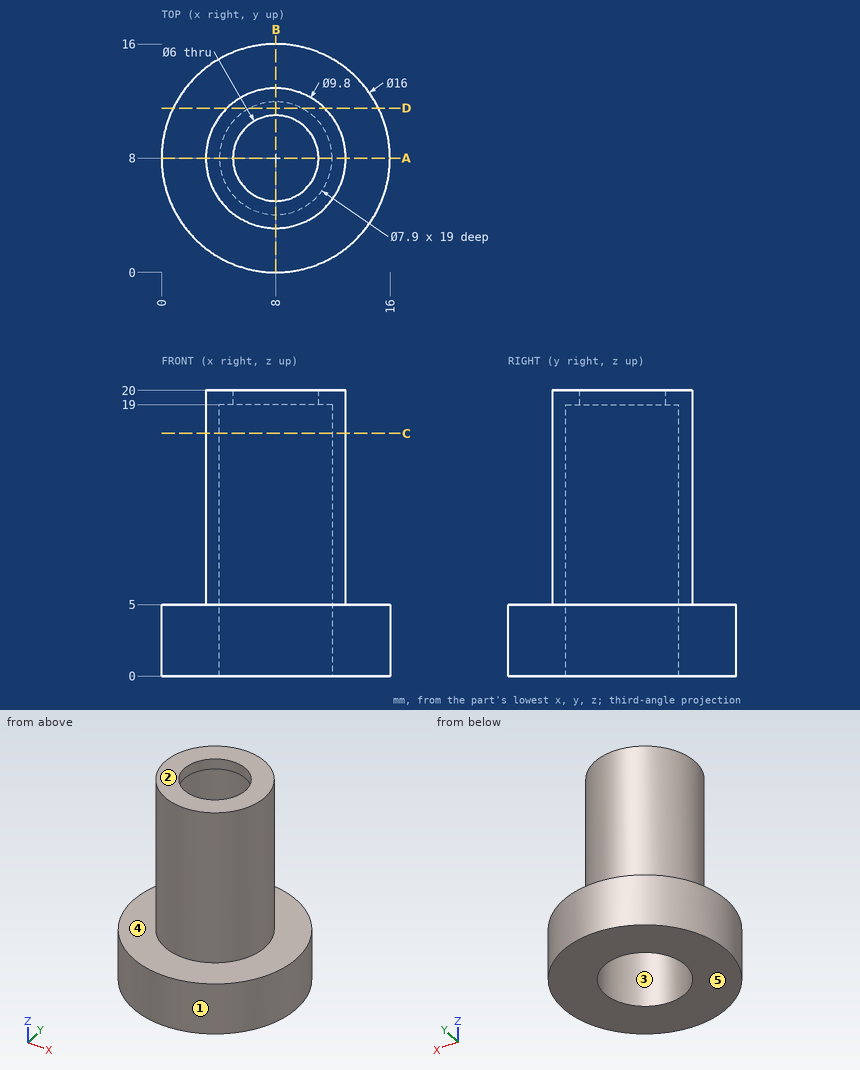
Drawing for the job (mm, zero at the part's lowest x, y, z). A direction names the side the tool comes from. Round coordinates to 2 decimals unless told otherwise and drop trailing zeros. Write each loop counter-clockwise with the first axis right and the second up, starting at its lowest first coordinate (ties: lowest second). Pieces come first, ordered by that corner, then holes.
Item 1: Band-saw the part on D-D on y = 11.5. Write the cut outline in (x, z), then the cut area to 3 significant figures.
Filled in:
outline: (0.81, 0) - (6.17, 0) - (6.17, 19) - (9.83, 19) - (9.83, 0) - (15.19, 0) - (15.19, 5) - (11.43, 5) - (11.43, 20) - (4.57, 20) - (4.57, 5) - (0.81, 5) - close
area: 105 mm2
Item 2: Drop flat-ended pins along their axis: pin 1 Ø5 at (y, z) = (3, 16) entering from -X; pin 2 Ø3 at (x, y) = (13, 13) entering from +Z; pin 3 Ø3.5 at (x, y) = (8, 8) entering from +Z; pin 4 Ø3 at (y, z) = (12.5, 15) entering from +X. Give the stop position or say it passes through.
Filled in:
pin 1: stops at x = 3.79
pin 2: stops at z = 5
pin 3: passes through
pin 4: stops at x = 11.87
Item 3: Tool access for the marked faces 4 and 5: list every direction of +Z, -Z, +X, -X, +Y, -Y with a clear straight run to the whole face (end or side of a thin tool).
Filled in:
face 4: +Z
face 5: -Z, +X, -X, +Y, -Y
Item 4: Mould opens along X. For the marked faces 1, 2 and 3 say: released by +X, released by -X, zero draft, split by the parting line, or undercut.
Filled in:
face 1: split by the parting line
face 2: zero draft
face 3: undercut
Item 5: Band-saw the part on A-A on y = 8. Write the cut outline in (x, z), then the cut area to 3 significant figures.
Filled in:
outline: (0, 0) - (4.05, 0) - (4.05, 19) - (5, 19) - (5, 20) - (3.1, 20) - (3.1, 5) - (0, 5) - close; (11, 19) - (11.95, 19) - (11.95, 0) - (16, 0) - (16, 5) - (12.9, 5) - (12.9, 20) - (11, 20) - close
area: 70.9 mm2
Item 6: Drill centre lines: L1, parallel to Y at x = 8, z = 13.5; L2, parallel to Y at x = 8, z = 19.55; L3, parallel to Z at x = 7, y = 1. Where is each one in solid material? Low to high.
Filled in:
L1: y = 3.1 to 4.05, 11.95 to 12.9
L2: y = 3.1 to 5, 11 to 12.9
L3: z = 0 to 5
Item 7: Band-saw the part on C-C on z = 17. Write the cut outline in (x, y).
Filled in:
outline: circle Ø9.8 at (8, 8); hole circle Ø7.9 at (8, 8)
